For this review, take the finished solid that the model builds, in its own axes (mm). Give positions to 0.01 mm unless a question says otherwise; leave off trailing zeros. Write each loop counter-clockwise with the first axis right and the second up, starting at its lowest first coordinate (ties: lowest second). Pieces come first, ordered by that corner, then holes.
1) For P1, Ø2, axis at x = 18.5, z = 25.5, coming from the -Y side; P2, Ø2, axis at y = 31.82, z = -31.82, coming from the -X side; P3, Ø6, axis at x = 22.5, z = -29, coming from the -Y side; P4, Ø3, axis at y = 16.77, z = 12.3, coming from the +X side, all flat-tipped, find the tip position at first contact; note any pin that passes through.
2) We need section A-A on y = 0. Give the boundary of the cut face in (x, z).
3) We need section D-D on y = -56. Give the boundary of the cut face in (x, z).
4) We need section B-B on x = 17.5. Give the number of separate pieces and of enclosed holes in the cut face, and give its area (3 significant figures).
5) Wall thickness on line 1 along Y through (x, z) = (17.5, 31.5); line 2 along Z through (x, y) = (17.75, -1); line 3 along Z through (x, y) = (16.5, 7): over which ranges is each line inside the solid? List them lowest first.
6) Draft analysis for pull direction Y (two halves, no side actions). For faces 1 (the face through (13.7, -1, -14)), 2 (the face through (19.78, -19.52, 62)), 3 (the face through (19.616, 22.938, 3.476)), state which applies: pulls with the +Y half, pulls with the -Y half, needs draft (parallel to the pull), parting line crosses it, or undercut.
7) We need section C-C on z = -40. Give the boundary of the cut face in (x, y), and give its area (3 significant figures).
from build123d import *

# Parameters (mm, degrees)
AXIAL_PROFILE_MM_W     = 12
AXIAL_PROFILE_MM_H     = 53.8875
AXIAL_HOLES_DEPTH      = 96.448886845
AXIAL_HOLES_DEPTH_BACK = 96.448886845
SKETCH2_R              = 2.4
CUT_EXTRUDE2_START     = 13.7
SKETCH3_R              = 1.25
CUT_EXTRUDE2_DEPTH     = 7


with BuildPart() as part:
    # Axial profile (mm) → Full revolution (revolve)
    with BuildSketch(Plane.XY, mode=Mode.PRIVATE) as full_revolution_sk:
        with Locations((19.7, 38.05625)):
            Rectangle(AXIAL_PROFILE_MM_W, AXIAL_PROFILE_MM_H)
    revolve(full_revolution_sk.sketch.rotate(Axis((-110, 0, 0), (1, 0, 0)), 90), axis=Axis((-110, 0, 0), (1, 0, 0)))

    # Sketch2 → Axial holes (cut, two sides: drawn at the far end of the back side and taken through both)
    with BuildSketch(Plane(origin=(0, 0, 0), x_dir=(0, 0, -1), z_dir=(1, 0, 0)).offset(-AXIAL_HOLES_DEPTH_BACK)):
        with Locations((-3.163812264, 20.557973926)):
            Circle(SKETCH2_R)
        with Locations((-12.299529665, 16.773835877)):
            Circle(SKETCH2_R)
    extrude(amount=AXIAL_HOLES_DEPTH + AXIAL_HOLES_DEPTH_BACK, mode=Mode.SUBTRACT)

    # Sketch3 → Cut-Extrude2 (cut)
    with BuildSketch(Plane(origin=(0, 0, 0), x_dir=(0, 0, -1), z_dir=(1, 0, 0)).offset(CUT_EXTRUDE2_START)):
        with Locations((-31.819805153, 31.819805153)):
            Circle(SKETCH3_R)
        with Locations((-31.819805153, -31.819805153)):
            Circle(SKETCH3_R)
        with Locations((31.819805153, -31.819805153)):
            Circle(SKETCH3_R)
        with Locations((31.819805153, 31.819805153)):
            Circle(SKETCH3_R)
    extrude(amount=CUT_EXTRUDE2_DEPTH, mode=Mode.SUBTRACT)


solid = part.part
Results list:
1. P1: stops at y = -60.21
1. P2: stops at x = 20.7
1. P3: stops at y = -59.57
1. P4: passes through
2. outline: (13.7, -65) - (25.7, -65) - (25.7, -11.11) - (13.7, -11.11) - close; (13.7, 11.11) - (25.7, 11.11) - (25.7, 65) - (13.7, 65) - close
3. outline: (13.7, -33) - (25.7, -33) - (25.7, 33) - (13.7, 33) - close
4. separate pieces: 1
4. enclosed holes: 7
4. area: 12,800 mm2
5. line 1: y = -56.86 to -33.03, -30.61 to 30.61, 33.03 to 56.86
5. line 2: z = -64.99 to -11.07, 11.07 to 64.99
5. line 3: z = -64.62 to -8.63, 8.63 to 64.62
6. face 1: needs draft
6. face 2: parting line crosses it
6. face 3: undercut
7. outline: (13.7, -51.23) - (25.7, -51.23) - (25.7, 51.23) - (13.7, 51.23) - close
7. area: 1,230 mm2
